Geometry check sheet. Reference: the model listing, model coordinates, mm. Face numbers are marked on the shaded views. A direction names the side the tool comes from. Round coordinates to 2 decimals unless told otherwise and drop trailing zeros. Write each loop counter-clockwise with the first axis right and the second up, starting at its lowest first coordinate (ties: lowest second). Pieces come first, ordered by that corner, then holes.
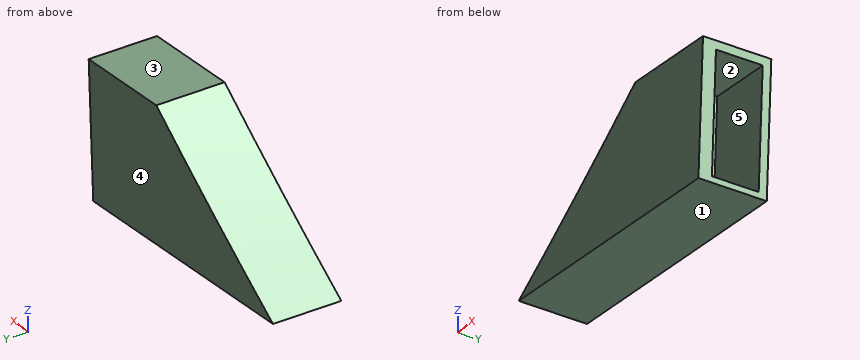
from build123d import *

# Parameters (mm, degrees)
BOSS_EXTRUDE2_DEPTH = 19
SKETCH3_W           = 33.25
SKETCH3_H           = 13
CUT_EXTRUDE2_DEPTH  = 19


with BuildPart() as part:
    # Sketch1 → Boss-Extrude2 (new body)
    with BuildSketch(Plane(origin=(0, 0, 0), x_dir=(1, 0, 0), z_dir=(0, 1, 0))):
        with BuildLine():
            Line((550.386370436, 820.819715378), (625.440328141, 824.647674335))
            Line((625.440328141, 824.647674335), (627.340180934, 787.397674335))
            Line((627.340180934, 787.397674335), (599.115957856, 785.958161072))
            ThreePointArc((599.115957856, 785.958161072), (575.015419514, 803.758315189), (550.386370436, 820.819715378))
        make_face()
    extrude(amount=BOSS_EXTRUDE2_DEPTH)

    # Sketch3 → Cut-Extrude2 (cut)
    with BuildSketch(Plane(origin=(665.767785772, 0, -33.955994289), x_dir=(-0.05093655241609126, 0, -0.9987018912708451), z_dir=(0.9987018912708452, 0, -0.05093655241609127))):
        with Locations((773.435764615, 10.189365534)):
            Rectangle(SKETCH3_W, SKETCH3_H)
    extrude(amount=-CUT_EXTRUDE2_DEPTH, mode=Mode.SUBTRACT)


solid = part.part
1. Depth check by flat-ended pin: pin 1 Ø4 at (y, z) = (7, -792.5) entering from -X; pin 2 Ø6 at (y, z) = (6.5, -809) entering from +X; pin 3 Ø1.5 at (x, y) = (612.5, 9) entering from +Z. Enter the tip coordinate at first touch or a pass-through.
2. Access from +Z, -Z, +X, -X, +Y, -Y to the whole of each face (thin tool, end or side, straight path). Record for the marked faces 1 and 2.
3. Section check A-A (y = 6). Record the cut outline in (x, z).
4. Section check D-D (y = 17.5). Record the cut outline in (x, z).
5. Section check C-C (x = 616). Record the cut outline in (y, z), plus the area to 3 significant figures.
6. Section check B-B (z = -802). Record the cut outline in (x, y), plus the area to 3 significant figures.
7. Release check for a two-part mould opening along Z. For the marked faces 3, 4 and 5 record: +Z half, -Z half, draft (parallel to the pull), parting line (faces both ways), or undercut.
8. Scan lines: line 1 along Y through (x, z) = (615.5, -815.5); line 2 along Z through (x, y) = (622, 7); line 3 along Z through (x, y) = (612.5, 8.75). Record each from-to range of solid material in increasing order.
Results below:
1. pin 1: stops at x = 587.74
1. pin 2: stops at x = 626.29
1. pin 3: stops at z = -786.6
2. face 1: -Z, -X, +Y, -Y
2. face 2: none
3. outline: (550.39, -820.82) - (625.44, -824.65) - (625.52, -822.99) - (606.55, -822.02) - (608.24, -788.82) - (627.22, -789.78) - (627.34, -787.4) - (599.12, -785.96) arc R988.27 cw to start
4. outline: (550.39, -820.82) - (625.44, -824.65) - (627.34, -787.4) - (599.12, -785.96) arc R988.27 cw to start
5. outline: (0, -824.17) - (19, -824.17) - (19, -786.82) - (0, -786.82) - close; hole (3.69, -822.51) - (16.69, -822.51) - (16.69, -789.21) - (3.69, -789.21) - close
5. area: 277 mm2
6. outline: (577.47, 0) - (626.6, 0) - (626.6, 3.69) - (607.57, 3.69) - (607.57, 16.69) - (626.6, 16.69) - (626.6, 19) - (577.47, 19) - close
6. area: 686 mm2
7. face 3: +Z half
7. face 4: draft
7. face 5: undercut
8. line 1: y = 0 to 3.69, 16.69 to 19
8. line 2: z = -824.47 to -822.81, -789.52 to -787.13
8. line 3: z = -823.99 to -822.33, -789.03 to -786.64
